Source: CAD feature listing. Evaluate the final solid. Frame: model axes, mm. Face numbers are marked on the shaded views. A direction names the side the tool comes from. Round coordinates to 2 decimals unless told otherwise and drop trailing zeros. Order: outer loops, then holes, each group sorted by start corner. A loop starts at its lowest first (then second) coordinate and runs counter-clockwise, first axis right, second up. Notation, with made-up numbers: (67.25, -5.5) - (82.25, -5.5) arc R8 ccw to (82.25, 5.5) - close; hole circle Ø7 at (38.25, -30.5). An arc over 180 degrees is marked (long way). Put each result on its own line as item: value. Start each with the question number.
1) Mould query, pull axis X, two halves, no side actions, for the marked faces 5, 6 and 7. Classes: +X half, -X half, draft (parallel to the pull), parting line (faces both ways), or undercut.
2) Section A-A on x = 0. Output: boundary loops of the cut face in (y, z).
3) Section B-B on y = -8.25. Output: boundary loops of the cut face in (x, z), then the cut area to 3 significant figures.
4) Access query for the marked faces 1, 2, 3 and 4. Directions: +Z, -Z, +X, -X, +Y, -Y. A direction counts if a zero-diameter tool reaches every point of the face in a straight line with its end or side. Return the directions, or none.
5) Contact query for flat-ended pins moving along their axis: P1, Ø2, axis at x = 1.5, y = -14, coming from the +Z side; P2, Ø8, axis at y = -14.5, z = -2.5, coming from the -X side; P3, Ø4.5, axis at x = -1.5, z = 2.5, coming from the +Y side; P4, Ø3.5, axis at x = 0.5, y = -11, coming from the -Z side. Output: stop coordinate, or through.
6) Line query: probe 1 along Y at (x, z) = (-1.5, 6.75); probe 2 along Z at (x, y) = (-2.5, -9.5); probe 3 along Z at (x, y) = (1.25, -14.5). Output: solid intervals per line, ascending. Write a range as [from, to].
7) Section C-C on z = 6. Output: boundary loops of the cut face in (x, y), then the cut area to 3 significant figures.
8) Section D-D on z = -0.5. Output: boundary loops of the cut face in (x, y), then the cut area to 3 significant figures.
Solid Edge part; units mm, degrees
sketch "Sketch1" plane through (0, 0, 0) normal (0, -1, 0) x (1, 0, 0)
  line L0 (-3.6639, 6.3461) -> (3.6639, 6.3461)
  line L1 (3.6639, 6.3461) -> (7.3279, 0)
  line L2 (7.3279, 0) -> (3.6639, -6.3461)
  line L3 (3.6639, -6.3461) -> (-3.6639, -6.3461)
  line L4 (-3.6639, -6.3461) -> (-7.3279, 0)
  line L5 (-7.3279, 0) -> (-3.6639, 6.3461)
extrude "Protrusion1" add sketch "Sketch1" along normal blind 20.32
sketch "Sketch2" plane through (0, 0, 0) normal (0, 1, 0) x (0.5, 0, -0.866)
  circle A0 centre (0, 0) radius 7.62
extrude "ExtrudedProtrusion_2" add sketch "Sketch2" along normal blind 1.5875
sketch "Sketch3" plane through (0, -20.32, 0) normal (0, -1, 0) x (-1, 0, 0)
  circle A0 centre (0, 0) radius 7.62
extrude "ExtrudedProtrusion_3" add sketch "Sketch3" along normal blind 1.5875
sketch "Sketch4" plane through (0, 1.5875, 0) normal (0, 1, 0) x (0, 0, 1)
  circle A0 centre (0, 0) radius 3
extrude "Cutout1" cut sketch "Sketch4" against normal up to next
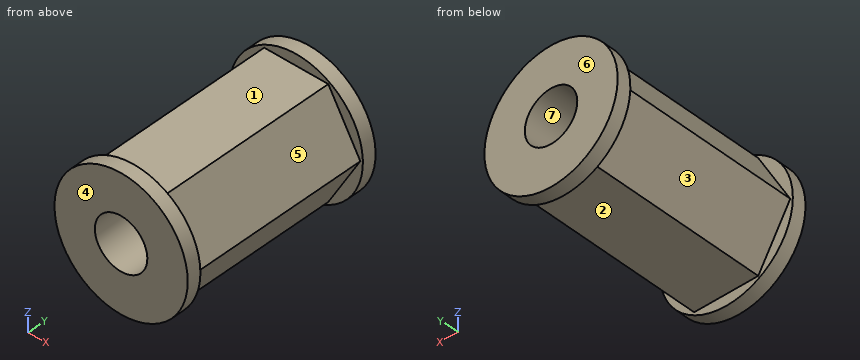
Answer sheet:
1. face 5: +X half
1. face 6: draft
1. face 7: undercut
2. outline: (-21.91, -7.62) - (-20.32, -7.62) - (-20.32, -6.35) - (0, -6.35) - (0, -7.62) - (1.59, -7.62) - (1.59, -3) - (-21.91, -3) - close; (-21.91, 3) - (1.59, 3) - (1.59, 7.62) - (0, 7.62) - (0, 6.35) - (-20.32, 6.35) - (-20.32, 7.62) - (-21.91, 7.62) - close
3. outline: (-7.33, 0) - (-3.66, -6.35) - (3.66, -6.35) - (7.33, 0) - (3.66, 6.35) - (-3.66, 6.35) - close; hole circle Ø6 at (0, 0)
3. area: 111 mm^2
4. face 1: +Z, +X, -X
4. face 2: -Z, +X, -X
4. face 3: -Z, -X
4. face 4: +Z, -Z, +X, -X, -Y
5. P1: z = 6.35
5. P2: x = -7.33
5. P3: y = 1.59
5. P4: z = -6.35
6. probe 1: [-21.91, -20.32], [0, 1.59]
6. probe 2: [-6.35, -1.66], [1.66, 6.35]
6. probe 3: [-6.35, -2.73], [2.73, 6.35]
7. outline: (-4.7, -21.91) - (4.7, -21.91) - (4.7, -20.32) - (3.86, -20.32) - (3.86, 0) - (4.7, 0) - (4.7, 1.59) - (-4.7, 1.59) - (-4.7, 0) - (-3.86, 0) - (-3.86, -20.32) - (-4.7, -20.32) - close
7. area: 187 mm^2
8. outline: (-7.6, -21.91) - (-2.96, -21.91) - (-2.96, 1.59) - (-7.6, 1.59) - (-7.6, 0) - (-7.04, 0) - (-7.04, -20.32) - (-7.6, -20.32) - close; (2.96, -21.91) - (7.6, -21.91) - (7.6, -20.32) - (7.04, -20.32) - (7.04, 0) - (7.6, 0) - (7.6, 1.59) - (2.96, 1.59) - close
8. area: 195 mm^2
